```python
from build123d import *

# Parameters (mm, degrees)
F1_R     = 10.9855
F2_DEPTH = 7


with BuildPart() as f2:
    # F1 (on Top) → F2 (new body)
    with BuildSketch(Plane.XY):
        Polygon((43.857164, 24.899659), (11.898966, 33.732012), (0, 50.871), (-11.898966, 33.732012), (-44.055578, 25.4355), (-35.162262, -6.561199), (-44.055578, -25.4355), (-23.263297, -27.170813), (0, -50.871), (23.263297, -27.170813), (44.055578, -25.4355), (35.162262, -6.561199), align=None)
        with Locations((-22.058533, -12.7355)):
            Circle(F1_R, mode=Mode.SUBTRACT)
        with Locations((22.058533, -12.7355)):
            Circle(F1_R, mode=Mode.SUBTRACT)
        Circle(F1_R, mode=Mode.SUBTRACT)
        with Locations((0, 25.471)):
            Circle(F1_R, mode=Mode.SUBTRACT)
    extrude(amount=F2_DEPTH)


solid = f2.part
```
Check sheet for the modelled part. Datum: model origin and axes. Units: mm. A direction names the side the tool comes from. Give positions to 0.01 mm unless a question says otherwise; leave off trailing zeros. Order: outer loops, then holes, each group sorted by start corner. A loop starts at its lowest first (then second) coordinate and runs counter-clockwise, first axis right, second up. Notation, with made-up numbers: M 61,69 L 103,69 A14 ccw 103,96 Z; hole C 67,-20 d9. An arc over 180 degrees is marked long. Answer in a Markdown table with one row per item. Add a question column.
Q1. Access from +Z, -Z, +X, -X, +Y, -Y to the whole of each face (thin tool, end or side, straight path). Record for faces 1 (the flat face through (11.469, -39.187, 3.451)), 2 (the flat face through (-39.55, -15.87, 3.45)), 3 (the flat face through (39.67, -16.13, 3.45)).
Q2. Sectioned sample at D-D, the plane x = -7. Record the boundary of the cut face in (y, z).
Q3. Sectioned sample at A-A, the plane x = 31.5. Record the boundary of the cut face in (y, z).
Q4. Sectioned sample at C-C, the plane z = 3.25. Record the boundary of the cut face in (x, y).
Q5. Gauge pin test, flat ends, axial feed: pin 1 Ø4 at (x, z) = (-3.5, 6) entering from +Y; pin 2 Ø1.5 at (y, z) = (-8, 4) entering from +X; pin 3 Ø4 at (x, z) = (28.5, 4.5) entering from -Y. Record the tip position at first contact, or that the pin passes through.
Q6. Release check for a two-part mould opening along X. For faces 4 (the cylindrical face through (32.206, -16.943, 3.451)), 5 (the flat face through (-27.752, 29.642, 3.451)), 6 (the flat face through (28.102, 29.254, 3.451)) record: released by +X, released by -X, zero draft, split by the parting line, or undercut.
Q7. Thickness scan on L1, parallel to Y at x = 0, z = 2.5; L2, parallel to Y at x = 0.5, z = 2.5; L3, parallel to X at y = -21, z = 3.75. Record the ranges inside material, lowest first.
Q8. Sectioned sample at B-B, the plane y = 27. Record the boundary of the cut face in (x, z).
Verdict:
| question | item | result |
|---|---|---|
| 1 | face 1 | +Z, -Z, +X, -Y |
| 1 | face 2 | +Z, -Z, -X |
| 1 | face 3 | +Z, -Z, +X |
| 2 | outline | M -43.74,0 L -8.47,0 L -8.47,7 L -43.74,7 Z; M 8.47,0 L 17,0 L 17,7 L 8.47,7 Z; M 33.94,0 L 40.79,0 L 40.79,7 L 33.94,7 Z |
| 3 | outline | M -26.48,0 L -18.35,0 L -18.35,7 L -26.48,7 Z; M -7.12,0 L 28.31,0 L 28.31,7 L -7.12,7 Z |
| 4 | outline | M -44.06,-25.44 L -23.26,-27.17 L 0,-50.87 L 23.26,-27.17 L 44.06,-25.44 L 35.16,-6.56 L 43.86,24.9 L 11.9,33.73 L 0,50.87 L -11.9,33.73 L -44.06,25.44 L -35.16,-6.56 Z; hole C -22.06,-12.74 d21.97; hole C 0,0 d21.97; hole C 0,25.47 d21.97; hole C 22.06,-12.74 d21.97 |
| 5 | pin 1 | y = 48.71 |
| 5 | pin 2 | x = 36.19 |
| 5 | pin 3 | y = -26.9 |
| 6 | face 4 | undercut |
| 6 | face 5 | released by -X |
| 6 | face 6 | released by +X |
| 7 | L1 | -50.87 to -10.99, 10.99 to 14.49, 36.46 to 50.87 |
| 7 | L2 | -50.36 to -10.97, 10.97 to 14.5, 36.45 to 50.15 |
| 7 | L3 | -41.97 to -29.3, -14.82 to 14.82, 29.3 to 41.97 |
| 8 | outline | M -37.99,0 L -10.88,0 L -10.88,7 L -37.99,7 Z; M 10.88,0 L 36.26,0 L 36.26,7 L 10.88,7 Z |
